from build123d import *

# Parameters (mm, degrees)
SKETCH1_R           = 9.5
BOSS_EXTRUDE1_DEPTH = 25
SKETCH2_R           = 5
CUT_EXTRUDE1_DEPTH  = 10
SKETCH3_R           = 2.5
CUT_EXTRUDE2_DEPTH  = 26


with BuildPart() as part:
    # Sketch1 → Boss-Extrude1 (new body)
    with BuildSketch(Plane(origin=(0, 0, 0), x_dir=(1, 0, 0), z_dir=(0, 1, 0))):
        Circle(SKETCH1_R)
    extrude(amount=BOSS_EXTRUDE1_DEPTH)

    # Sketch2 → Cut-Extrude1 (cut)
    with BuildSketch(Plane.XZ):
        Circle(SKETCH2_R)
    extrude(amount=-CUT_EXTRUDE1_DEPTH, mode=Mode.SUBTRACT)

    # Sketch3 → Cut-Extrude2 (cut, through all)
    with BuildSketch(Plane(origin=(0, 25, 0), x_dir=(1, 0, 0), z_dir=(0, 1, 0))):
        Circle(SKETCH3_R)
    extrude(amount=-CUT_EXTRUDE2_DEPTH, mode=Mode.SUBTRACT)


solid = part.part
For this review, take the finished solid that the model builds, in its own axes (mm). A direction names the side the tool comes from. Give positions to 0.01 mm unless a question says otherwise; leave off trailing zeros. Loops run counter-clockwise (first coordinate to the right, second up) from the corner with the lowest first, then second, coordinate; pieces in that order, holes last. Notation, with made-up numbers: (41, -17.75) - (95, -17.75) arc R15 ccw to (95, 3.25) - close; hole circle Ø9 at (-20.5, 4). An arc over 180 degrees is marked (long way). Write each question's results on one line, items separated by ' | '.
(1) Take a section at C-C (y = 15.75). Give the boundary of the cut face in (x, z), then the cut area to 3 significant figures.
Conclusion:
outline: circle Ø19 at (0, 0); hole circle Ø5 at (0, 0) | area: 264 mm^2
(2) For faces 4 (the flat face through (2, 10, -2)), 5 (the flat face through (2, 25, 2)), list the 3-axis set-ups (+Z, -Z, +X, -X, +Y, -Y) from which the entire face can be reached by the end or side of a thin tool; tool diameter is ignored.
Conclusion:
face 4: -Y | face 5: +Z, -Z, +X, -X, +Y
(3) Take a section at B-B (z = 0). Give the boundary of the cut face in (x, y).
Conclusion:
outline: (-9.5, 0) - (-5, 0) - (-5, 10) - (-2.5, 10) - (-2.5, 25) - (-9.5, 25) - close; (2.5, 10) - (5, 10) - (5, 0) - (9.5, 0) - (9.5, 25) - (2.5, 25) - close
(4) Take a section at D-D (z = -3.75). Give the boundary of the cut face in (x, y), then the cut area to 3 significant figures.
Conclusion:
outline: (-8.73, 0) - (-3.31, 0) - (-3.31, 10) - (3.31, 10) - (3.31, 0) - (8.73, 0) - (8.73, 25) - (-8.73, 25) - close | area: 370 mm^2
(5) For line 1 along X through (y, z) = (16.25, 0); line 2 along Z through (x, y) = (0, 6.25), list the stretches that pass through material, from the lowest coordinate up.
Conclusion:
line 1: -9.5 to -2.5, 2.5 to 9.5 | line 2: -9.5 to -5, 5 to 9.5
(6) Take a section at A-A (x = 0). Give the boundary of the cut face in (y, z).
Conclusion:
outline: (0, -9.5) - (25, -9.5) - (25, -2.5) - (10, -2.5) - (10, -5) - (0, -5) - close; (0, 5) - (10, 5) - (10, 2.5) - (25, 2.5) - (25, 9.5) - (0, 9.5) - close
(7) Draft analysis for pull direction Z (two halves, no side actions). For faces 1 (the cylindrical face through (4.38, 12.32, 8.43)), 2 (the cylindrical face through (-1.08, 4.93, -4.88)), 3 (the flat face through (4, 0, 4)), state which applies: +Z half, -Z half, draft (parallel to the pull), parting line (faces both ways), or undercut.
Conclusion:
face 1: parting line | face 2: undercut | face 3: draft
(8) For pin 1 Ø4 at (y, z) = (20.5, 1) entering from +X; pin 2 Ø2 at (x, z) = (2.5, -1) entering from -Y; pin 3 Ø1 at (y, z) = (12.5, 3) entering from +X; pin 4 Ø1 at (x, y) = (-1, 7.5) entering from -Z, all flat-tipped, find the tip position at first contact; note any pin that passes through.
Conclusion:
pin 1: x = 9.5 | pin 2: y = 10 | pin 3: x = 9.17 | pin 4: z = -9.49
